Design review of the part built by this model. Coordinates are the model's own, in mm. Give positions to 0.01 mm unless a question says otherwise; leave off trailing zeros. Loops run counter-clockwise (first coordinate to the right, second up) from the corner with the lowest first, then second, coordinate; pieces in that order, holes last. Notation, with made-up numbers: M -38.75,-22 L 16.25,-22 A20 cw 16.25,6 Z; hole C -27,-19 d6. An arc over 180 degrees is marked long. Use a Markdown table: item, result. Add a question column.
(1) Add section C-C, the plane z = 0.85. State how many separate pieces and enclosed holes the cut face has, then the cut area to 3 significant figures.
(2) Add section B-B, the plane x = 52.5. Give the boundary of the cut face in (y, z), then the cut area to 3 significant figures.
(3) Insertion check: pin 1 Ø5 at (x, y) = (263.5, -39.5) entering from -Z; pin 2 Ø1.5 at (x, z) = (53.5, 1) entering from -Y; pin 3 Ø1 at (x, z) = (138, 1) entering from -Y; pin 4 Ø1.5 at (x, z) = (148, 1) entering from +Y. Each pin has a flat end and moves straight along its axis. Give the tip position at first contact, or say it passes through.
(4) Add section D-D, the plane x = 126. Give the boundary of the cut face in (y, z), then the cut area to 3 significant figures.
(5) Add section A-A, the plane y = -172.5. Give the boundary of the cut face in (x, z), then the cut area to 3 significant figures.
(6) Draft analysis for pull direction X (two halves, no side actions). For faces 1 (the face through (201.12, -35.175, 1.479)), 2 (the face through (267, -178, 1)), 3 (the face through (150, -96, 0)), state which applies: pulls with the +X half, pulls with the -X half, needs draft (parallel to the pull), parting line crosses it, or undercut.
(7) For probe 1 along X at (y, z) = (-97.5, 2.5); probe 2 along Y at (x, z) = (278, 2.85); probe 3 along X at (y, z) = (-40.5, 0.4), list the stretches that pass through material, from the lowest coordinate up.
```python
from build123d import *

# Parameters (mm, degrees)
ESQUISSE1_R        = 2.75
ESQUISSE1_R_2      = 11
ESQUISSE1_R_3      = 1.5
ESQUISSE1_W        = 7
ESQUISSE1_H        = 50
BOSS_EXTRU_1_DEPTH = 3


with BuildPart() as part:
    # Esquisse1 → Boss.-Extru.1 (new body)
    with BuildSketch(Plane.XY):
        with BuildLine():
            Line((5, 0), (41.684938398, 0))
            ThreePointArc((41.684938398, 0), (44.389031178, -0.794303597), (46.23397571, -2.924847105))
            ThreePointArc((46.23397571, -2.924847105), (93.045262331, -35.129096737), (143.5, -9))
            Line((143.5, -9), (151.5, -9))
            ThreePointArc((151.5, -9), (201.954737669, -35.129096737), (248.76602429, -2.924847105))
            ThreePointArc((248.76602429, -2.924847105), (250.610968822, -0.794303597), (253.315061602, 0))
            Line((253.315061602, 0), (290, 0))
            ThreePointArc((290, 0), (293.535533906, -1.464466094), (295, -5))
            Line((295, -5), (295, -190))
            ThreePointArc((295, -190), (293.535533906, -193.535533906), (290, -195))
            Line((290, -195), (253.315061602, -195))
            ThreePointArc((253.315061602, -195), (250.610968822, -194.205696403), (248.76602429, -192.075152895))
            ThreePointArc((248.76602429, -192.075152895), (201.954737669, -159.870903263), (151.5, -186))
            Line((151.5, -186), (143.5, -186))
            ThreePointArc((143.5, -186), (93.045262331, -159.870903263), (46.23397571, -192.075152895))
            ThreePointArc((46.23397571, -192.075152895), (44.389031178, -194.205696403), (41.684938398, -195))
            Line((41.684938398, -195), (5, -195))
            ThreePointArc((5, -195), (1.464466094, -193.535533906), (0, -190))
            Line((0, -190), (0, -5))
            ThreePointArc((0, -5), (1.464466094, -1.464466094), (5, 0))
        make_face()
        with Locations((60, -40)):
            Circle(ESQUISSE1_R, mode=Mode.SUBTRACT)
        with Locations((17, -17.00000759)):
            Circle(ESQUISSE1_R_2, mode=Mode.SUBTRACT)
        with Locations((6, -6.00000759)):
            Circle(ESQUISSE1_R_3, mode=Mode.SUBTRACT)
        with Locations((28, -6.00000759)):
            Circle(ESQUISSE1_R_3, mode=Mode.SUBTRACT)
        with Locations((28, -28.00000759)):
            Circle(ESQUISSE1_R_3, mode=Mode.SUBTRACT)
        with Locations((6, -28.00000759)):
            Circle(ESQUISSE1_R_3, mode=Mode.SUBTRACT)
        with Locations((235, -40)):
            Circle(ESQUISSE1_R, mode=Mode.SUBTRACT)
        with Locations((289, -6.00000759)):
            Circle(ESQUISSE1_R_3, mode=Mode.SUBTRACT)
        with Locations((267, -6.00000759)):
            Circle(ESQUISSE1_R_3, mode=Mode.SUBTRACT)
        with Locations((278, -17.00000759)):
            Circle(ESQUISSE1_R_2, mode=Mode.SUBTRACT)
        with Locations((289, -28.00000759)):
            Circle(ESQUISSE1_R_3, mode=Mode.SUBTRACT)
        with Locations((267, -28.00000759)):
            Circle(ESQUISSE1_R_3, mode=Mode.SUBTRACT)
        with Locations((267, -188.99999241)):
            Circle(ESQUISSE1_R_3, mode=Mode.SUBTRACT)
        with Locations((289, -188.99999241)):
            Circle(ESQUISSE1_R_3, mode=Mode.SUBTRACT)
        with Locations((289, -166.99999241)):
            Circle(ESQUISSE1_R_3, mode=Mode.SUBTRACT)
        with Locations((267, -166.99999241)):
            Circle(ESQUISSE1_R_3, mode=Mode.SUBTRACT)
        with Locations((278, -177.99999241)):
            Circle(ESQUISSE1_R_2, mode=Mode.SUBTRACT)
        with Locations((235, -155)):
            Circle(ESQUISSE1_R, mode=Mode.SUBTRACT)
        with Locations((60, -155)):
            Circle(ESQUISSE1_R, mode=Mode.SUBTRACT)
        with Locations((6, -188.99999241)):
            Circle(ESQUISSE1_R_3, mode=Mode.SUBTRACT)
        with Locations((28, -188.99999241)):
            Circle(ESQUISSE1_R_3, mode=Mode.SUBTRACT)
        with Locations((17, -177.99999241)):
            Circle(ESQUISSE1_R_2, mode=Mode.SUBTRACT)
        with Locations((6, -166.99999241)):
            Circle(ESQUISSE1_R_3, mode=Mode.SUBTRACT)
        with Locations((28, -166.99999241)):
            Circle(ESQUISSE1_R_3, mode=Mode.SUBTRACT)
        with BuildLine():
            Line((228, -77.5), (228, -117.5))
            ThreePointArc((228, -117.5), (229.464466094, -121.035533906), (233, -122.5))
            Line((233, -122.5), (253, -122.5))
            ThreePointArc((253, -122.5), (256.535533906, -121.035533906), (258, -117.5))
            Line((258, -117.5), (258, -77.5))
            ThreePointArc((258, -77.5), (256.535533906, -73.964466094), (253, -72.5))
            Line((253, -72.5), (233, -72.5))
            ThreePointArc((233, -72.5), (229.464466094, -73.964466094), (228, -77.5))
        make_face(mode=Mode.SUBTRACT)
        with BuildLine():
            Line((42, -72.5), (62, -72.5))
            ThreePointArc((62, -72.5), (65.535533906, -73.964466094), (67, -77.5))
            Line((67, -77.5), (67, -117.5))
            ThreePointArc((67, -117.5), (65.535533906, -121.035533906), (62, -122.5))
            Line((62, -122.5), (42, -122.5))
            ThreePointArc((42, -122.5), (38.464466094, -121.035533906), (37, -117.5))
            Line((37, -117.5), (37, -77.5))
            ThreePointArc((37, -77.5), (38.464466094, -73.964466094), (42, -72.5))
        make_face(mode=Mode.SUBTRACT)
        with Locations((286, -97.5)):
            Rectangle(ESQUISSE1_W, ESQUISSE1_H, mode=Mode.SUBTRACT)
        with Locations((9, -97.5)):
            Rectangle(ESQUISSE1_W, ESQUISSE1_H, mode=Mode.SUBTRACT)
    extrude(amount=BOSS_EXTRU_1_DEPTH)


solid = part.part
```
Established:
| question | item | result |
|---|---|---|
| 1 | separate pieces | 1 |
| 1 | enclosed holes | 28 |
| 1 | area | 41,500 mm^2 |
| 2 | outline | M -181.59,0 L -122.5,0 L -122.5,3 L -181.59,3 Z; M -72.5,0 L -13.41,0 L -13.41,3 L -72.5,3 Z |
| 2 | area | 355 mm^2 |
| 3 | pin 1 | z = 0 |
| 3 | pin 2 | y = -181.27 |
| 3 | pin 3 | y = -179.14 |
| 3 | pin 4 | y = -9 |
| 4 | outline | M -168.31,0 L -26.69,0 L -26.69,3 L -168.31,3 Z |
| 4 | area | 425 mm^2 |
| 5 | outline | M 0,0 L 7.47,0 L 7.47,3 L 0,3 Z; M 26.53,0 L 61.21,0 L 61.21,3 L 26.53,3 Z; M 131.77,0 L 163.23,0 L 163.23,3 L 131.77,3 Z; M 233.79,0 L 268.47,0 L 268.47,3 L 233.79,3 Z; M 287.53,0 L 295,0 L 295,3 L 287.53,3 Z |
| 5 | area | 347 mm^2 |
| 6 | face 1 | undercut |
| 6 | face 2 | undercut |
| 6 | face 3 | needs draft |
| 7 | probe 1 | 0 to 5.5, 12.5 to 37, 67 to 228, 258 to 282.5, 289.5 to 295 |
| 7 | probe 2 | -195 to -189, -167 to -28, -6 to 0 |
| 7 | probe 3 | 0 to 57.3, 62.7 to 232.3, 237.7 to 295 |
